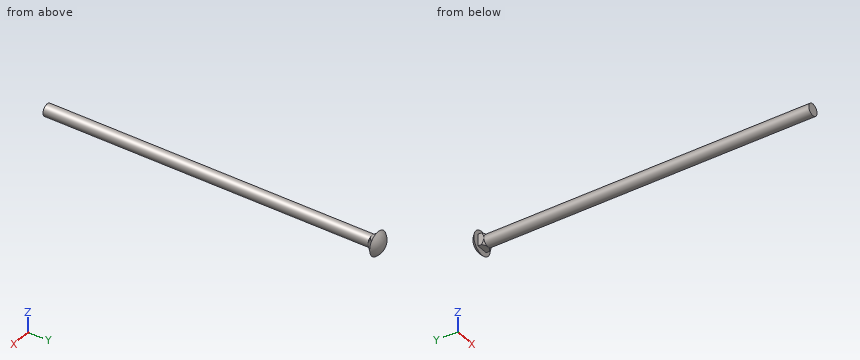
from build123d import *

# Parameters (mm, degrees)
SKETCH1_R           = 6.35
BOSS_EXTRUDE1_DEPTH = 349.25
SKETCH2_W           = 12.7
SKETCH2_H           = 12.7
BOSS_EXTRUDE2_DEPTH = 6.35
SKETCH3_R           = 12.7
BOSS_EXTRUDE3_DEPTH = 6.35
SKETCH5_OUTSIDE_W   = 112.846
SKETCH5_OUTSIDE_H   = 112.846
SKETCH5_OUTSIDE_R   = 6.35
CUT_EXTRUDE1_DEPTH  = 6.35
CUT_EXTRUDE1_TAPER  = 45


with BuildPart() as part:
    # Sketch1 → Boss-Extrude1 (new body)
    with BuildSketch(Plane(origin=(0, 0, 0), x_dir=(1, 0, 0), z_dir=(0, 1, 0))):
        Circle(SKETCH1_R)
    extrude(amount=BOSS_EXTRUDE1_DEPTH)

    # Sketch2 → Boss-Extrude2 (add)
    with BuildSketch(Plane(origin=(0, 349.25, 0), x_dir=(1, 0, 0), z_dir=(0, 1, 0))):
        Rectangle(SKETCH2_W, SKETCH2_H)
    extrude(amount=BOSS_EXTRUDE2_DEPTH)

    # Sketch3 → Boss-Extrude3 (add)
    with BuildSketch(Plane(origin=(0, 355.6, 0), x_dir=(1, 0, 0), z_dir=(0, 1, 0))):
        Circle(SKETCH3_R)
    extrude(amount=BOSS_EXTRUDE3_DEPTH)

    # Sketch4 → Cut-Revolve1 (revolve, cut)
    with BuildSketch(Plane(origin=(0, 0, 0), x_dir=(0, 0, -1), z_dir=(1, 0, 0))):
        with BuildLine():
            Line((-12.7, 355.6), (-17.199061604, 355.6))
            Line((-17.199061604, 355.6), (-17.199061604, 364.492507037))
            Line((-17.199061604, 364.492507037), (0, 364.492507037))
            Line((0, 364.492507037), (0, 361.95))
            ThreePointArc((0, 361.95), (-7.099515829, 360.274031657), (-12.7, 355.6))
        make_face()
    revolve(axis=Axis((0, 369.557753648, 0), (0, -1, 0)), mode=Mode.SUBTRACT)

    # Sketch5 outside → Cut-Extrude1 (cut)
    with BuildSketch(Plane.XZ.offset(-349.25)):
        Rectangle(SKETCH5_OUTSIDE_W, SKETCH5_OUTSIDE_H)
        Circle(SKETCH5_OUTSIDE_R, mode=Mode.SUBTRACT)
    extrude(amount=-CUT_EXTRUDE1_DEPTH, taper=CUT_EXTRUDE1_TAPER, mode=Mode.SUBTRACT)


solid = part.part
Can you work these out from the model? Positions are in its coordinate system, mm. Give positions to 0.01 mm unless a question says otherwise; leave off trailing zeros. Loops run counter-clockwise (first coordinate to the right, second up) from the corner with the lowest first, then second, coordinate; pieces in that order, holes last. Notation, with made-up numbers: (-15, 2) -> (34, 2) arc R36 cw to (34, 40) -> close; hole circle Ø11 at (60.5, -8.5). An arc over 180 degrees is marked (long way). Write item = value, one per line.
1) Will these pins go through, and if not, where does the flat tip stop? pin 1 (3 mm diameter, centred on x = -1, y = 352, fed in from +Z); pin 2 (3 mm diameter, centred on y = 205.5, z = 4, fed in from +X); pin 3 (3 mm diameter, centred on y = 353, z = 2.5, fed in from -X).
Check result:
pin_1 = 6.35
pin_2 = 5.84
pin_3 = -6.35
2) Suppose I cut it at A-A on y = 111. Write out the boundary of the cut face in (x, z).
Check result:
outline = circle Ø12.7 at (0, 0)
3) I need wall thicknesses on L1, parallel to Y at x = -1.5, z = 0.75; L2, parallel to Y at x = 6.25, z = 3; L3, parallel to Z at x = 4, y = 100.5. Which ranges of each line are inside material? Lowest first, please. Write a range as from..to.
Check result:
L1 = 0..361.86
L2 = 349.83..360.36
L3 = -4.93..4.93
